Check sheet for the modelled part. Datum: model origin and axes. Units: mm. Face numbers are marked on the shaded views. Coordinates: 2 decimals unless noted, no trailing zeros. Loops run counter-clockwise (first coordinate to the right, second up) from the corner with the lowest first, then second, coordinate; pieces in that order, holes last.
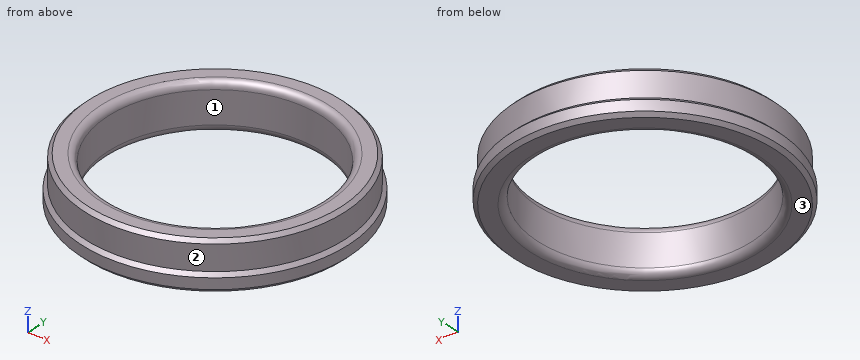
from build123d import *

# Parameters (mm, degrees)
SKETCH1_R           = 37.5
SKETCH1_R_2         = 30.05
BOSS_EXTRUDE1_DEPTH = 5
SKETCH2_R           = 36.5
SKETCH2_R_2         = 30.05
BOSS_EXTRUDE2_DEPTH = 8
CHAMFER1_SIZE       = 1
FILLET1_R           = 2


with BuildPart() as part:
    # Sketch1 → Boss-Extrude1 (new body)
    with BuildSketch(Plane.XY):
        Circle(SKETCH1_R)
        Circle(SKETCH1_R_2, mode=Mode.SUBTRACT)
    extrude(amount=BOSS_EXTRUDE1_DEPTH)

    # Sketch2 → Boss-Extrude2 (add)
    with BuildSketch(Plane.XY.offset(5)):
        Circle(SKETCH2_R)
        Circle(SKETCH2_R_2, mode=Mode.SUBTRACT)
    extrude(amount=BOSS_EXTRUDE2_DEPTH)

    # Chamfer1
    chamfer1_edges = [part.edges().sort_by_distance(p)[0] for p in [
        (-36.5, 0, 13),
        (-37.5, 0, 0),
        (-37.5, 0, 5),
    ]]
    chamfer(chamfer1_edges, length=CHAMFER1_SIZE - 0.0001)  # a hair under: the kernel refuses the full size

    # Fillet1
    fillet1_edges = [part.edges().sort_by_distance(p)[0] for p in [
        (-30.05, 0, 13),
        (-30.05, 0, 0),
    ]]
    fillet(fillet1_edges, radius=FILLET1_R)


solid = part.part
(1) Scan lines: line 1 along Y through (x, z) = (0, 8.25); line 2 along X through (y, z) = (23, 3.5); line 3 along Y through (x, z) = (-7.5, 8). Record each from-to range of solid material in increasing order.
(2) Gauge pin test, flat ends, axial feed: P1, Ø1, axis at x = -26, z = 8.5, coming from the +Y side; P2, Ø3, axis at x = 16.5, z = 4, coming from the -Y side; P3, Ø1, axis at y = 0.5, z = 8.5, coming from the +X side. Record the tip position at first contact, or that the pin passes through.
(3) Section check C-C, the plane z = 6.75. Enter the section's corners in (x, y).
(4) Draft check along Y on the marked faces 1, 2 and 3. Enter one of: pulls with the +Y half, pulls with the -Y half, needs draft (parallel to the pull), parting line crosses it, or undercut.
Determined:
1. line 1: y = -36.5 to -30.05, 30.05 to 36.5
1. line 2: x = -29.62 to -19.34, 19.34 to 29.62
1. line 3: y = -35.72 to -29.1, 29.1 to 35.72
2. P1: stops at y = 26.12
2. P2: stops at y = -34.37
2. P3: stops at x = 36.5
3. outline: circle Ø73 at (0, 0); hole circle Ø60.1 at (0, 0)
4. face 1: undercut
4. face 2: parting line crosses it
4. face 3: needs draft
